from build123d import *

# Parameters (mm, degrees)
F1_DEPTH = 20
F2_R     = 1.5
F3_DEPTH = 20
F4_W     = 2.8
F4_H     = 6
F5_DEPTH = 7.5
F6_R     = 2.25
F7_DEPTH = 6


with BuildPart() as f1:
    # F0 (on Top) → F1 (new body)
    with BuildSketch(Plane.XY):
        with BuildLine():
            Line((-38.333333, 9.652778), (-38.333333, -5.347222))
            Line((-38.333333, -5.347222), (-18.333333, -5.347222))
            Line((-18.333333, -5.347222), (-18.333333, 9.652778))
            Line((-18.333333, 9.652778), (-27.583333, 9.652778))
            Line((-27.583333, 9.652778), (-27.583333, 3.683597))
            ThreePointArc((-27.583333, 3.683597), (-25.18016, 2.273369), (-24.233333, -0.347222))
            ThreePointArc((-24.233333, -0.347222), (-30.953925, -3.500395), (-29.083333, 3.683597))
            Line((-29.083333, 3.683597), (-29.083333, 9.652778))
            Line((-29.083333, 9.652778), (-38.333333, 9.652778))
        make_face()
        Polygon((-48.333333, -5.347222), (-48.333333, -11.347222), (-8.333333, -11.347222), (-8.333333, -5.347222), (-18.333333, -5.347222), (-38.333333, -5.347222), align=None)
    extrude(amount=F1_DEPTH)

    # F2 (on face) → F3 (cut)
    with BuildSketch(Plane(origin=(-38.333333, 0, 0), x_dir=(0, -1, 0), z_dir=(-1, 0, 0))):
        with Locations((-6.152778, 10)):
            Circle(F2_R)
    extrude(amount=-F3_DEPTH, mode=Mode.SUBTRACT)

    # F4 (on face) → F5 (cut)
    with BuildSketch(Plane(origin=(0, 9.652778, 0), x_dir=(-1, 0, 0), z_dir=(0, 1, 0))):
        with Locations((20.733333, 10)):
            Rectangle(F4_W, F4_H)
    extrude(amount=-F5_DEPTH, mode=Mode.SUBTRACT)

    # F6 (on face) → F7 (cut)
    with BuildSketch(Plane(origin=(0, -5.347222, 0), x_dir=(-1, 0, 0), z_dir=(0, 1, 0))):
        with Locations((43.333333, 10)):
            Circle(F6_R)
        with Locations((13.333333, 10)):
            Circle(F6_R)
    extrude(amount=-F7_DEPTH, mode=Mode.SUBTRACT)


solid = f1.part
Input: part model. Units: mm. Frame: model coordinates. A direction names the side the tool comes from. Coordinates: 2 decimals unless noted, no trailing zeros. Loops run counter-clockwise (first coordinate to the right, second up) from the corner with the lowest first, then second, coordinate; pieces in that order, holes last. Notation, with made-up numbers: (16, -37.5) - (33, -37.5) arc R13 cw to (33, -21.5) - close; hole circle Ø10 at (67, 50.5). An arc over 180 degrees is marked (long way). Answer in a Markdown table with one row per item. Add a question column.
Item 1: Access query for faces 4 (the flat face through (-38.333, 2, 10)), 5 (the flat face through (-29.083, 8, 10)), 6 (the flat face through (-18.333, 2, 10)), 7 (the flat face through (-22.133, 5.1, 8.6)). Directions: +Z, -Z, +X, -X, +Y, -Y. A direction counts if a zero-diameter tool reaches every point of the face in a straight line with its end or side. Return the directions, or none.
Item 2: Section query A-A on x = -37. Return the cut outline in (y, z), then the cut area to 3 significant figures.
Item 3: Line query: line 1 along X through (y, z) = (6, 16); line 2 along Z through (x, y) = (-13.5, -6.75); line 3 along Z through (x, y) = (-37.5, 6.25). Output: solid intervals per line, ascending. Write a range as [from, to].
Item 4: Section query B-B on y = 6. Return the cut outline in (x, z).
Item 5: Contact query for flat-ended pins moving along their axis: P1, Ø3, axis at x = -12.5, z = 7, coming from the +Y side; P2, Ø11, axis at x = -41.5, z = 10.5, coming from the +Y side; P3, Ø12, axis at y = 1, z = 5.5, coming from the +X side; P4, Ø6.5, axis at y = 5.5, z = 11.5, coming from the -X side. Output: stop coordinate, or through.
Item 6: Mould query, pull axis Z, two halves, no side actions, for faces 1 (the flat face through (-29, -5, 0)), 2 (the flat face through (-34, 9.653, 10)), 3 (the cylindrical face through (-24.896, 4.767, 9.425)). Classes: released by +Z, released by -Z, zero draft, split by the parting line, or undercut.
Item 7: Section query D-D on x = -26. Return the cut outline in (y, z).
Item 8: Section query C-C on z = 10. State how many separate pieces and enclosed holes the cut face has, then the cut area to 3 significant figures.
Recorded:
| question | item | result |
|---|---|---|
| 1 | face 4 | +Z, -Z, -X, +Y |
| 1 | face 5 | +Z, -Z, +Y |
| 1 | face 6 | +Z, -Z, +X, +Y |
| 1 | face 7 | +Y |
| 2 | outline | (-11.35, 0) - (9.65, 0) - (9.65, 20) - (-11.35, 20) - close; hole circle Ø3 at (6.15, 10) |
| 2 | area | 413 mm^2 |
| 3 | line 1 | [-38.33, -29.08], [-27.58, -18.33] |
| 3 | line 2 | [0, 7.76], [12.24, 20] |
| 3 | line 3 | [0, 8.5], [11.5, 20] |
| 4 | outline | (-38.33, 0) - (-29.08, 0) - (-29.08, 8.51) - (-38.33, 8.51) - close; (-38.33, 11.49) - (-29.08, 11.49) - (-29.08, 20) - (-38.33, 20) - close; (-27.58, 0) - (-18.33, 0) - (-18.33, 8.51) - (-19.33, 8.51) - (-19.33, 7) - (-22.13, 7) - (-22.13, 8.51) - (-27.58, 8.51) - close; (-27.58, 11.49) - (-22.13, 11.49) - (-22.13, 13) - (-19.33, 13) - (-19.33, 11.49) - (-18.33, 11.49) - (-18.33, 20) - (-27.58, 20) - close |
| 5 | P1 | y = -5.35 |
| 5 | P2 | y = 9.65 |
| 5 | P3 | x = -18.33 |
| 5 | P4 | x = -38.33 |
| 6 | face 1 | released by -Z |
| 6 | face 2 | zero draft |
| 6 | face 3 | undercut |
| 7 | outline | (-11.35, 0) - (-3.72, 0) - (-3.72, 20) - (-11.35, 20) - close; (3.02, 0) - (9.65, 0) - (9.65, 20) - (3.02, 20) - close; hole circle Ø3 at (6.15, 10) |
| 8 | separate pieces | 6 |
| 8 | enclosed holes | 0 |
| 8 | area | 356 mm^2 |
